Check sheet for the modelled part. Datum: model origin and axes. Units: mm. Round coordinates to 2 decimals unless told otherwise and drop trailing zeros. Write each loop counter-clockwise with the first axis right and the second up, starting at its lowest first coordinate (ties: lowest second). Pieces come first, ordered by that corner, then holes. Notation, with made-up numbers: (33.5, 48.5) -> (92.5, 48.5) arc R26 cw to (92.5, 83.5) -> close; hole circle Ø8 at (33.25, -21.75). An arc over 180 degrees is marked (long way). One line per item, written item: value.
Autodesk Fusion 360 part; units mm, degrees
sketch "Sketch2" plane through (0, 0, 0) normal (0, 1, 0) x (1, 0, 0)
  circle A0 centre (0, 0) radius 3.5
  circle A1 centre (0, 0) radius 9.5
  circle A2 centre (0, 0) radius 20
  circle A3 centre (0, 0) radius 14
  line L0 (0, 9.5) -> (0, 14)
  line L1 (-1.5, 13.9194) -> (-1.5, 9.3808)
  line L2 (1.5, 13.9194) -> (1.5, 9.3808)
  dimension "d5" = 7
  dimension "d6" = 6
  dimension "d7" = 40
  dimension "d8" = 6
  dimension "d11" = 1.5
  dimension "d12" = 1.5
extrude "Extrude3" add sketch "Sketch2" along normal blind 116 contours A1 A3 L0 L2 | A1 A3 L0 L1 makes body 1
extrude "Extrude2" add sketch "Sketch2" along normal blind 116 separate body contours A1 | A2 makes body 2 at (9.4528, 38.6667, 0.9459) makes body 3 at (19.9751, 77.3333, 0.9969)
pattern_circular "C-Pattern1" count 6 over 360 about axis through (0, 1.75, 0) along (0, 1, 0) of bodies 1 makes body 4 at (-9.9944, 38.6667, -7.5023) makes body 5 at (-11.4944, 38.6667, 4.9042) makes body 6 at (-1.5, 38.6667, 12.4066) makes body 7 at (9.9944, 38.6667, 7.5023) makes body 8 at (9.9944, 38.6667, -7.5023)
combine "Combine1" operation add target body 1 tool bodies 2 3 7 8 4 5 6
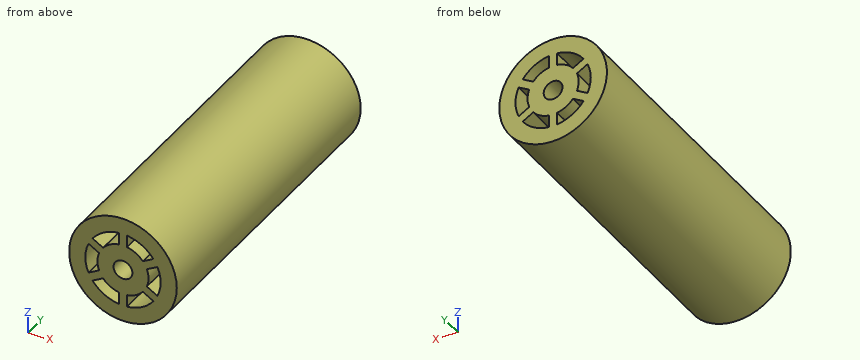
Item 1: Sectioned sample at A-A on x = 0. Enter the section's corners in (y, z).
Answer:
outline: (0, -20) -> (116, -20) -> (116, -3.5) -> (0, -3.5) -> close; (0, 3.5) -> (116, 3.5) -> (116, 20) -> (0, 20) -> close
Item 2: Thickness scan on line 1 (X direction, y = 74.5, z = 0); line 2 (Z direction, x = 0, y = 30); line 3 (X direction, y = 57, z = -12). Record the ranges inside material, lowest first.
Answer:
line 1: x = -20 to -14, -9.5 to -3.5, 3.5 to 9.5, 14 to 20
line 2: z = -20 to -3.5, 3.5 to 20
line 3: x = -16 to -7.21, -1.5 to 1.5, 7.21 to 16
Item 3: Sectioned sample at D-D on z = -15.5. Enter the section's corners in (x, y).
Answer:
outline: (-12.64, 0) -> (12.64, 0) -> (12.64, 116) -> (-12.64, 116) -> close
Item 4: Sectioned sample at C-C on y = 35. Enter the section's corners in (x, z), and give its area (3 significant figures).
Answer:
outline: circle Ø40 at (0, 0); hole (-12.8, -5.66) -> (-8.87, -3.39) arc R9.5 cw to (-8.87, 3.39) -> (-12.8, 5.66) arc R14 ccw to start; hole (-11.3, -8.26) arc R14 ccw to (-1.5, -13.92) -> (-1.5, -9.38) arc R9.5 cw to (-7.37, -5.99) -> close; hole (-11.3, 8.26) -> (-7.37, 5.99) arc R9.5 cw to (-1.5, 9.38) -> (-1.5, 13.92) arc R14 ccw to start; hole circle Ø7 at (0, 0); hole (1.5, -13.92) arc R14 ccw to (11.3, -8.26) -> (7.37, -5.99) arc R9.5 cw to (1.5, -9.38) -> close; hole (1.5, 9.38) arc R9.5 cw to (7.37, 5.99) -> (11.3, 8.26) arc R14 ccw to (1.5, 13.92) -> close; hole (8.87, -3.39) -> (12.8, -5.66) arc R14 ccw to (12.8, 5.66) -> (8.87, 3.39) arc R9.5 cw to start
area: 967 mm^2
Item 5: Sectioned sample at B-B on z = 0. Enter the section's corners in (x, y).
Answer:
outline: (-20, 0) -> (-14, 0) -> (-14, 116) -> (-20, 116) -> close; (-9.5, 0) -> (-3.5, 0) -> (-3.5, 116) -> (-9.5, 116) -> close; (3.5, 0) -> (9.5, 0) -> (9.5, 116) -> (3.5, 116) -> close; (14, 0) -> (20, 0) -> (20, 116) -> (14, 116) -> close
Item 6: Depth check by flat-ended pin: P1, Ø12, axis at x = 15.5, y = 17, coming from the +Z side; P2, Ø2, axis at x = -6.5, z = 13.5, coming from the -Y side; P3, Ø1.4, axis at y = 36.5, z = 11.5, coming from the -X side; P4, Ø10, axis at x = 4, y = 77, coming from the -Z side. Enter the tip coordinate at first touch or a pass-through.
Answer:
P1: stops at z = 17.6
P2: stops at y = 0
P3: stops at x = -16.83
P4: stops at z = -20
